```python
from build123d import *

# Parameters (mm, degrees)
SKETCH1_R           = 3.25
BOSS_EXTRUDE1_DEPTH = 36
SKETCH2_R           = 2.6
CUT_EXTRUDE1_DEPTH  = 4.2
CUT_EXTRUDE3_DEPTH  = 7
CUT_EXTRUDE2_DEPTH  = 24
SKETCH6_R           = 3.25
BOSS_EXTRUDE2_DEPTH = 0.4
CHAMFER1_SIZE       = 1


with BuildPart() as part:
    # Sketch1 → Boss-Extrude1 (new body)
    with BuildSketch(Plane.XY):
        with BuildLine():
            Line((-14.75, -7.4), (-14.75, -11.5))
            Line((-14.75, -11.5), (-23.75, -11.5))
            Line((-23.75, -11.5), (-23.75, -7.4))
            ThreePointArc((-23.75, -7.4), (-21.675125708, -3.893735462), (-17.603054495, -4.025))
            ThreePointArc((-17.603054495, -4.025), (-13.947306078, -1.606859229), (-18.188386592, -0.5))
            ThreePointArc((-18.188386592, -0.5), (-25.210418213, 1.109132257), (-19.583771133, 5.607918465))
            ThreePointArc((-19.583771133, 5.607918465), (-17.193366172, 5.79117644), (-16.154186894, 7.951668465))
            ThreePointArc((-16.154186894, 7.951668465), (-12.264338175, 12.248774426), (-8.166591783, 8.149443113))
            ThreePointArc((-8.166591783, 8.149443113), (-7.324900269, 6.763678693), (-5.714627865, 6.952915098))
            ThreePointArc((-5.714627865, 6.952915098), (0, 9), (5.714627865, 6.952915098))
            ThreePointArc((5.714627865, 6.952915098), (7.324900269, 6.763678693), (8.166591783, 8.149443113))
            ThreePointArc((8.166591783, 8.149443113), (12.264338175, 12.248774426), (16.154186894, 7.951668465))
            ThreePointArc((16.154186894, 7.951668465), (17.193366172, 5.79117644), (19.583771133, 5.607918465))
            ThreePointArc((19.583771133, 5.607918465), (25.210418213, 1.109132257), (18.188386592, -0.5))
            ThreePointArc((18.188386592, -0.5), (13.947306078, -1.606859229), (17.603054495, -4.025))
            ThreePointArc((17.603054495, -4.025), (21.675125708, -3.893735462), (23.75, -7.4))
            Line((23.75, -7.4), (23.75, -11.5))
            Line((23.75, -11.5), (14.75, -11.5))
            Line((14.75, -11.5), (14.75, -7.4))
            Line((14.75, -7.4), (21.583030278, -7.4))
            ThreePointArc((21.583030278, -7.4), (21.980389985, -7.203488489), (22.065406667, -6.768421053))
            ThreePointArc((22.065406667, -6.768421053), (20.615569602, -5.16152077), (18.461832697, -5.375))
            ThreePointArc((18.461832697, -5.375), (12.368918668, -1.344765382), (19.437386192, 0.5))
            ThreePointArc((19.437386192, 0.5), (23.650605164, 1.465479354), (20.274616916, 4.164751079))
            ThreePointArc((20.274616916, 4.164751079), (16.290608649, 4.470181037), (14.558643186, 8.071001079))
            ThreePointArc((14.558643186, 8.071001079), (12.359417834, 10.642138999), (9.774460347, 8.459173783))
            Line((9.774460347, 8.459173783), (8.965752283, -0.784401685))
            ThreePointArc((8.965752283, -0.784401685), (0, -9), (-8.965752283, -0.784401685))
            Line((-8.965752283, -0.784401685), (-9.774460347, 8.459173783))
            ThreePointArc((-9.774460347, 8.459173783), (-12.359417834, 10.642138999), (-14.558643186, 8.071001079))
            ThreePointArc((-14.558643186, 8.071001079), (-16.290608649, 4.470181037), (-20.274616916, 4.164751079))
            ThreePointArc((-20.274616916, 4.164751079), (-23.650605164, 1.465479354), (-19.437386192, 0.5))
            ThreePointArc((-19.437386192, 0.5), (-12.368918668, -1.344765382), (-18.461832697, -5.375))
            ThreePointArc((-18.461832697, -5.375), (-20.615569602, -5.16152077), (-22.065406667, -6.768421053))
            ThreePointArc((-22.065406667, -6.768421053), (-21.980389985, -7.203488489), (-21.583030278, -7.4))
            Line((-21.583030278, -7.4), (-14.75, -7.4))
        make_face()
        Circle(SKETCH1_R, mode=Mode.SUBTRACT)
    extrude(amount=BOSS_EXTRUDE1_DEPTH)

    # Sketch2 → Cut-Extrude1 (cut)
    with BuildSketch(Plane.XZ.offset(11.5)):
        with Locations(Location((-19.225, 30.5, 0), (0, 0, 270))):  # turned: the seam where the file's is
            Circle(SKETCH2_R)
        with Locations(Location((-19.225, 5.5, 0), (0, 0, 270))):  # turned: the seam where the file's is
            Circle(SKETCH2_R)
        with Locations(Location((19.225, 5.5, 0), (0, 0, 270))):  # turned: the seam where the file's is
            Circle(SKETCH2_R)
        with Locations(Location((19.225, 30.5, 0), (0, 0, 270))):  # turned: the seam where the file's is
            Circle(SKETCH2_R)
    extrude(amount=-CUT_EXTRUDE1_DEPTH, mode=Mode.SUBTRACT)

    # Sketch5 → Cut-Extrude3 (cut)
    with BuildSketch(Plane.XY):
        Polygon((5.25, -3.031088913), (5.25, 3.031088913), (0, 6.062177826), (-5.25, 3.031088913), (-5.25, -3.031088913), (0, -6.062177826), align=None)
    extrude(amount=CUT_EXTRUDE3_DEPTH, mode=Mode.SUBTRACT)

    # Sketch3 → Cut-Extrude2 (cut)
    with BuildSketch(Plane.XY.offset(36)):
        Polygon((5.25, -3.031088913), (5.25, 3.031088913), (0, 6.062177826), (-5.25, 3.031088913), (-5.25, -3.031088913), (0, -6.062177826), align=None)
    extrude(amount=-CUT_EXTRUDE2_DEPTH, mode=Mode.SUBTRACT)

    # Sketch6 → Boss-Extrude2 (add)
    with BuildSketch(Plane(origin=(0, 0, 7), x_dir=(-1, 0, 0), z_dir=(0, 0, -1))):
        Circle(SKETCH6_R)
    extrude(amount=-BOSS_EXTRUDE2_DEPTH)

    # Chamfer1
    chamfer1_edges = [part.edges().sort_by_distance(p)[0] for p in [
        (2.625, -4.54663337, 0),
        (5.25, 0, 0),
        (2.625, 4.54663337, 0),
        (-2.625, 4.54663337, 0),
        (-5.25, 0, 0),
        (-2.625, -4.54663337, 0),
    ]]
    chamfer(chamfer1_edges, length=CHAMFER1_SIZE)


solid = part.part
```
Input: part model. Units: mm. Frame: model coordinates. A direction names the side the tool comes from. Give positions to 0.01 mm unless a question says otherwise; leave off trailing zeros. Order: outer loops, then holes, each group sorted by start corner. A loop starts at its lowest first (then second) coordinate and runs counter-clockwise, first axis right, second up. Notation, with made-up numbers: M 18.5,46 L 37.5,46 A26 ccw 37.5,82 Z; hole C 55.25,71.5 d11. An arc over 180 degrees is marked long. One line per question, with ' | ' between items. Start each with the question number.
1. Section query B-B (z = 5.5). Count the separate pieces of the cut face and the enclosed holes in it, and give its area (3 significant figures).
2. Section query C-C (x = 15.5). Return the cut outline in (y, z), and give its area (3 significant figures).
3. Pull-direction query (Y, two-part tool) for faces 1 (the face through (0, 9, 18)), 2 (the face through (-9.364, 3.773, 17.748)), 3 (the face through (2.828, -4.999, 0.507)), 4 (the face through (-25.18, 0.99, 17.75)); classes: released by +Y, released by -Y, zero draft, split by the parting line, or undercut.
4. Section query A-A (x = -21). Return the cut outline in (y, z).
5. Access query for faces 5 (the face through (-23.75, -9, 18)), 6 (the face through (0, 0, 7)), 7 (the face through (0, 0, 7.4)). Directions: +Z, -Z, +X, -X, +Y, -Y. A direction counts if a zero-diameter tool reaches every point of the face in a straight line with its end or side. Return the directions, or none.
6. First-contact query: pin 1 Ø1.8 at (y, z) = (-0.5, 5) entering from -X; pin 2 Ø3 at (x, z) = (19.225, 5.5) entering from -Y; pin 3 Ø4.5 at (x, z) = (19.225, 30.5) entering from -Y; pin 4 Ø6 at (x, z) = (14, 30.5) entering from -Y. Flat tips, straight axial feed; report the tip coordinate or a pass-through.
7. Material intervals for probe 1 along X at (y, z) = (-9.75, 5.5) (3 decimals); probe 2 along Y at (x, z) = (-20, 13.5); probe 3 along Y at (x, z) = (0, 28.5), sorted ascending. Write a range as [from, to].
Here are the results:
1) separate pieces: 3 | enclosed holes: 1 | area: 382 mm²
2) outline: M -11.5,0 L -7.4,0 L -7.4,36 L -11.5,36 Z; M -5.92,0 L -4.26,0 L -4.26,36 L -5.92,36 Z; M 0.26,0 L 1.92,0 L 1.92,36 L 0.26,36 Z; M 5.18,0 L 10.46,0 L 10.46,36 L 5.18,36 Z | area: 457 mm²
3) face 1: released by +Y | face 2: released by -Y | face 3: undercut | face 4: undercut
4) outline: M -11.5,0 L -7.4,0 L -7.4,3.6 L -11.5,3.6 Z; M -11.5,7.4 L -7.4,7.4 L -7.4,28.6 L -11.5,28.6 Z; M -11.5,32.4 L -7.4,32.4 L -7.4,36 L -11.5,36 Z; M -5.35,0 L -3.6,0 L -3.6,36 L -5.35,36 Z; M -1.99,0 L -0.38,0 L -0.38,36 L -1.99,36 Z; M 4.38,0 L 5.99,0 L 5.99,36 L 4.38,36 Z
5) face 5: +Z, -Z, -X, -Y | face 6: -Z | face 7: +Z
6) pin 1: x = -24.98 | pin 2: y = -5.74 | pin 3: y = -5.95 | pin 4: y = -11.5
7) probe 1: [-23.75, -21.825], [-16.625, -14.75], [14.75, 16.625], [21.825, 23.75] | probe 2: [-11.5, -7.4], [-5.01, -3.41], [-1.78, -0.01], [4.05, 5.78] | probe 3: [-9, -6.06], [6.06, 9]
